from build123d import *

# Parameters (mm, degrees)
CUT_EXTRUDE6_DEPTH = 10


with BuildPart() as part:
    # Sketch1 → Revolve2 (revolve)
    with BuildSketch(Plane.XY):
        with BuildLine():
            Line((0, 6.102087539), (0, -3.366129571))
            Line((0, -3.366129571), (0, -4.366129571))
            Line((0, -4.366129571), (-2, -4.366129571))
            Line((-2, -4.366129571), (-2, -3.366129571))
            Line((-2, -3.366129571), (-3, -3.366129571))
            Line((-3, -3.366129571), (-3, 3.633870429))
            Line((-3, 3.633870429), (-5, 3.633870429))
            Line((-5, 3.633870429), (-5, 5.633870429))
            ThreePointArc((-5, 5.633870429), (-3.134722719, 6.735016577), (-1, 7.102087539))
            Line((-1, 7.102087539), (-1, 6.102087539))
            Line((-1, 6.102087539), (0, 6.102087539))
        make_face()
    revolve(axis=Axis((0, 6.102087539, 0), (0, -1, 0)))

    # Sketch2 → Cut-Extrude6 (cut)
    with BuildSketch(Plane.ZY.offset(5)):
        Polygon((-1, 7.153918726), (-1, 7.78774413), (1, 7.78774413), (1, 7.102087539), (1, 5.633870429), (-1, 5.633870429), (-1, 7.102087539), align=None)
    extrude(amount=-CUT_EXTRUDE6_DEPTH, mode=Mode.SUBTRACT)


solid = part.part
Model file for the job. Use its own axes, mm. A direction names the side the tool comes from. Give positions to 0.01 mm unless a question says otherwise; leave off trailing zeros. Order: outer loops, then holes, each group sorted by start corner. A loop starts at its lowest first (then second) coordinate and runs counter-clockwise, first axis right, second up. Notation, with made-up numbers: M 46,73.5 L 56,73.5 A17 cw 56,79.5 Z; hole C -15.75,19.25 d4. An arc over 180 degrees is marked long. Write item = value, one per line.
Q1. Drill centre lines: line 1 (Y direction, x = 1.75, z = 0.5); line 2 (Y direction, x = -2.75, z = 0.75); line 3 (Z direction, x = 2, y = 6.5). Where is each one in solid material? Low to high. Write a range as [from, to].
Derived:
line_1 = [-4.37, 5.63]
line_2 = [-3.37, 5.63]
line_3 = [-3.1, -1], [1, 3.1]
Q2. Cut at A-A, the plane z = 0. List the corners of the cut face in (x, y).
Derived:
outline = M -5,3.63 L -3,3.63 L -3,-3.37 L -2,-3.37 L -2,-4.37 L 2,-4.37 L 2,-3.37 L 3,-3.37 L 3,3.63 L 5,3.63 L 5,5.63 L -5,5.63 Z
Q3. Flat gauge pins, fed straight in: pin 1 (0.7 mm diameter, centred on x = 1.5, y = 6, fed in from +Z); pin 2 (5 mm diameter, centred on x = -3.5, z = 0, fed in from +Y); pin 3 (2 mm diameter, centred on y = 4.5, z = -3.5, fed in from +X); pin 4 (5 mm diameter, centred on y = 2, z = 0.5, fed in from +X). Where does each tip first touch, or does it go through?
Derived:
pin_1 = 4.76
pin_2 = 7.08
pin_3 = 4.33
pin_4 = 5
Q4. Cut at B-B, the plane y = -2.75. List the corners of the cut face in (x, z).
Derived:
outline = C 0,0 d6
Q5. Two-plate mould, pull along Z, no slides. Class faces 4 (the flat face through (1, -3.366, 2)), 5 (the flat face through (0, 5.634, 0)), 6 (the cylindrical face through (0, -4, 2)): pulls with the +Z half, pulls with the -Z half, needs draft (parallel to the pull), parting line crosses it, or undercut.
Derived:
face_4 = needs draft
face_5 = undercut
face_6 = parting line crosses it
Q6. Tool access for faces 1 (the cylindrical face through (1.08, 4.65, 4.88)), 2 (the flat face through (0, 6, -1)), 3 (the flat face through (3.3, 3.634, -0.1)): list every direction of +Z, -Z, +X, -X, +Y, -Y with a clear straight run to the whole face (end or side of a thin tool).
Derived:
face_1 = +Y, -Y
face_2 = +X, -X, +Y
face_3 = -Y
